Work out the finished part from the listing and answer in its coordinate system (mm). Face numbers are marked on the shaded views. Coordinates: 2 decimals unless noted, no trailing zeros. Order: outer loops, then holes, each group sorted by start corner. A loop starts at its lowest first (then second) coordinate and runs counter-clockwise, first axis right, second up. Notation, with made-up numbers: (57.25, -36.75) -> (96.25, -36.75) arc R7 cw to (96.25, -27.75) -> close; hole circle Ø10 at (-24, 73). An arc over 180 degrees is marked (long way). Answer as CSV lines item,"result". Start each with the question number.
Item 1: Section C-C (z = 4.5) is taken. Write down the section's boundary in (x, y), then the cut area to 3 significant figures.
Item 2: Each of these flat-tipped pins is pushed along its axis until it touches: pin 1 Ø6.5 at (x, y) = (15.11, 50.57) entering from -Z; pin 2 Ø3 at (x, y) = (-15.5, -50.5) entering from +Z. Where does it stop, or does it pass through?
Item 3: Section A-A (y = 9.5) is taken. Write down the section's boundary in (x, z), then the cut area to 3 significant figures.
Item 4: Straight lines are drawn through the part: L1, parallel to Y at x = -15.5, z = 6; L2, parallel to Y at x = -16.5, z = 7.75; L3, parallel to Y at x = 11, z = 5. For each, find the intervals that lie inside material, in ascending order.
Item 5: Section B-B (x = -6.5) is taken. Write down the section's boundary in (y, z).
Item 6: For a pull along X with two mould halves and no side action, classify the marked faces 1, 2, 3 and 4 as pulls with the +X half, pulls with the -X half, needs draft (parallel to the pull), parting line crosses it, or undercut.
```python
from build123d import *

# Parameters (mm, degrees)
F0_W     = 38
F0_H     = 108
F0_R     = 2
F1_DEPTH = 9
F2_R     = 3


with BuildPart() as f1:
    # F0 (on Top) → F1 (new body)
    with BuildSketch(Plane.XY):
        with BuildLine():
            ThreePointArc((5.706968, -5.714822), (7.712615, -8.087528), (8.791989, -11.000826))
            ThreePointArc((8.791989, -11.000826), (11.232354, -10.554221), (12.600096, -12.624032))
            ThreePointArc((12.600096, -12.624032), (11.232354, -14.693844), (8.791989, -14.247239))
            ThreePointArc((8.791989, -14.247239), (7.713498, -17.159023), (5.709659, -19.530996))
            ThreePointArc((5.709659, -19.530996), (8.425965, -20.996255), (10.784891, -22.986424))
            ThreePointArc((10.784891, -22.986424), (13.862215, -18.206159), (14.939576, -12.624032))
            ThreePointArc((14.939576, -12.624032), (13.862843, -7.043472), (10.787222, -2.264082))
            ThreePointArc((10.787222, -2.264082), (8.425588, -4.252233), (5.706968, -5.714822))
        make_face()
        with BuildLine():
            ThreePointArc((-8.919726, -11.038862), (-7.830592, -8.082615), (-5.789315, -5.682866))
            ThreePointArc((-5.789315, -5.682866), (-8.499762, -4.205185), (-10.850307, -2.203935))
            ThreePointArc((-10.850307, -2.203935), (-15.060422, -12.616237), (-10.861132, -23.032909))
            ThreePointArc((-10.861132, -23.032909), (-8.510775, -21.032627), (-5.800788, -19.555715))
            ThreePointArc((-5.800788, -19.555715), (-7.814796, -17.19237), (-8.905782, -14.285245))
            ThreePointArc((-8.905782, -14.285245), (-12.720827, -12.678409), (-8.919726, -11.038862))
        make_face()
        with BuildLine():
            ThreePointArc((5.603682, 1.265457), (8.381963, -0.225399), (10.787222, -2.264082))
            ThreePointArc((10.787222, -2.264082), (13.905039, 2.536774), (14.997339, 8.156016))
            ThreePointArc((14.997339, 8.156016), (13.878906, 13.839509), (10.690392, 18.675455))
            ThreePointArc((10.690392, 18.675455), (8.324534, 16.666348), (5.595827, 15.187174))
            ThreePointArc((5.595827, 15.187174), (7.57988, 12.907076), (8.697198, 10.09871))
            ThreePointArc((8.697198, 10.09871), (11.379114, 10.5015), (12.850096, 8.223097))
            ThreePointArc((12.850096, 8.223097), (11.379114, 5.944693), (8.697198, 6.347483))
            ThreePointArc((8.697198, 6.347483), (7.582521, 3.543455), (5.603682, 1.265457))
        make_face()
        with BuildLine():
            ThreePointArc((-10.842957, 18.523657), (-15.00266, 8.161334), (-10.850307, -2.203935))
            ThreePointArc((-10.850307, -2.203935), (-8.49497, -0.220064), (-5.784132, 1.241002))
            ThreePointArc((-5.784132, 1.241002), (-7.772737, 3.510479), (-8.899446, 6.309695))
            ThreePointArc((-8.899446, 6.309695), (-13.060362, 8.167454), (-8.915558, 10.060887))
            ThreePointArc((-8.915558, 10.060887), (-7.810312, 12.874025), (-5.83607, 15.162624))
            ThreePointArc((-5.83607, 15.162624), (-8.510157, 16.588935), (-10.842957, 18.523657))
        make_face()
        Rectangle(F0_W, F0_H)
        with Locations((-15.5, -50.5)):
            Circle(F0_R, mode=Mode.SUBTRACT)
        with BuildLine():
            ThreePointArc((14.997339, 8.156016), (13.905039, 2.536774), (10.787222, -2.264082))
            ThreePointArc((10.787222, -2.264082), (13.862843, -7.043472), (14.939576, -12.624032))
            ThreePointArc((14.939576, -12.624032), (13.862215, -18.206159), (10.784891, -22.986424))
            ThreePointArc((10.784891, -22.986424), (13.894801, -27.783287), (14.984183, -33.3953))
            ThreePointArc((14.984183, -33.3953), (-5.597944, -47.317938), (-10.861132, -23.032909))
            ThreePointArc((-10.861132, -23.032909), (-15.060422, -12.616237), (-10.850307, -2.203935))
            ThreePointArc((-10.850307, -2.203935), (-15.00266, 8.161334), (-10.842957, 18.523657))
            ThreePointArc((-10.842957, 18.523657), (-5.833397, 42.924664), (14.850096, 29.043097))
            ThreePointArc((14.850096, 29.043097), (13.771383, 23.457599), (10.690392, 18.675455))
            ThreePointArc((10.690392, 18.675455), (13.878906, 13.839509), (14.997339, 8.156016))
        make_face(mode=Mode.SUBTRACT)
        with Locations((15.107894, -50.56573)):
            Circle(F0_R, mode=Mode.SUBTRACT)
        with Locations((-15.5, 50.5)):
            Circle(F0_R, mode=Mode.SUBTRACT)
        with Locations((15.107894, 50.56573)):
            Circle(F0_R, mode=Mode.SUBTRACT)
    extrude(amount=F1_DEPTH)

    # F2
    f2_edges = [f1.edges().sort_by_distance(p)[0] for p in [
        (19, 54, 4.5),
        (19, -54, 4.5),
        (-19, -54, 4.5),
        (-19, 54, 4.5),
    ]]
    fillet(f2_edges, radius=F2_R)


solid = f1.part
```
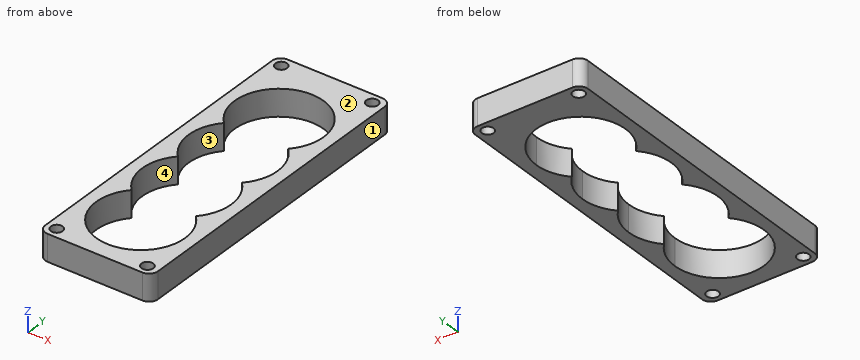
Checked values:
1,outline,"(-19, -51) arc R3 ccw to (-16, -54) -> (16, -54) arc R3 ccw to (19, -51) -> (19, 51) arc R3 ccw to (16, 54) -> (-16, 54) arc R3 ccw to (-19, 51) -> close; hole circle Ø4 at (-15.5, -50.5); hole circle Ø4 at (-15.5, 50.5); hole (-10.86, -23.03) arc R15 ccw (long way) to (14.98, -33.4) arc R15 ccw to (10.78, -22.99) arc R15 ccw to (14.94, -12.62) arc R15 ccw to (10.79, -2.26) arc R15 ccw to (15, 8.16) arc R15 ccw to (10.69, 18.68) arc R15 ccw to (14.85, 29.04) arc R15 ccw (long way) to (-10.84, 18.52) arc R15 ccw to (-10.85, -2.2) arc R15 ccw to start; hole circle Ø4 at (15.11, -50.57); hole circle Ø4 at (15.11, 50.57)"
1,area,"1,630 mm^2"
2,pin 1,"stops at z = 0"
2,pin 2,"passes through"
3,outline,"(-19, 0) -> (-14.94, 0) -> (-14.94, 9) -> (-19, 9) -> close; (14.94, 0) -> (19, 0) -> (19, 9) -> (14.94, 9) -> close"
3,area,"73.1 mm^2"
4,L1,"y = -54 to -52.5, -48.5 to 48.5, 52.5 to 54"
4,L2,"y = -53.96 to -52.23, -48.77 to 48.77, 52.23 to 53.96"
4,L3,"y = -54 to -43.58, -23.21 to -22.76, -2.49 to -2.04, 18.35 to 19.01, 39.08 to 54"
5,outline,"(-54, 0) -> (-46.92, 0) -> (-46.92, 9) -> (-54, 9) -> close; (42.63, 0) -> (54, 0) -> (54, 9) -> (42.63, 9) -> close"
6,face 1,"pulls with the +X half"
6,face 2,"needs draft"
6,face 3,"undercut"
6,face 4,"undercut"
